Read the model definition and answer for the solid it produces. Units are mm, in the model's axes. Give positions to 0.01 mm unless a question says otherwise; leave off trailing zeros. Loops run counter-clockwise (first coordinate to the right, second up) from the corner with the lowest first, then second, coordinate; pieces in that order, holes last. Notation, with made-up numbers: (68, -23.5) - (75, -23.5) arc R29 cw to (75, 15.5) - close; hole circle Ø2 at (-18, 70). An arc over 180 degrees is marked (long way). Write each question's results on one line, items separated by ' | '. Start each with the question number.
Q1. The part is cut by section A-A, the plane x = -114.5. Write down the section's boundary in (y, z), plus the area to 3 significant figures.
Q2. Find the intervals of material crossed by line 1 (Y direction, x = -215.5, z = 2.7); line 2 (X direction, y = 172.5, z = 1.9); line 3 (Y direction, x = -101, z = 3.9), in increasing order. Write a range as from..to.
Q3. Given pin 1 (1.8 mm diameter, centred on y = 336, z = 3.5, fed in from -X); pin 2 (1.8 mm diameter, centred on x = -61, z = 3.5, fed in from -Y); pin 3 (3 mm diameter, centred on y = 123.5, z = 1.5, fed in from +X), each flat-ended and moving along its own axis, determine where each tip first touches the part or whether it passes through.
Q4. The part is cut by section B-B, the plane z = 1.8. State how many separate pieces and enclosed holes the cut face has, plus the area to 3 significant figures.
Q5. The part is cut by section D-D, the plane y = 53.5. Write down the section's boundary in (x, z), plus the area to 3 significant figures.
Q6. The part is cut by section C-C, the plane x = -172.5. Write down the section's boundary in (y, z), plus the area to 3 significant figures.
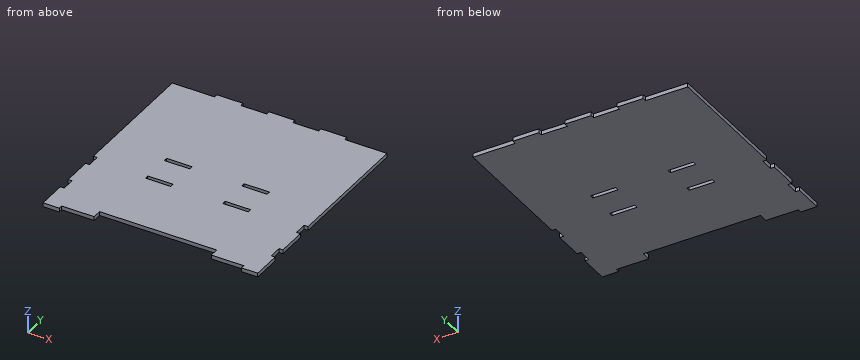
```python
from build123d import *

# Parameters (mm, degrees)
ESQUISSE1_W             = 330
ESQUISSE1_H             = 340
BOSS_EXTRU_1_DEPTH      = 6
ESQUISSE2_W             = 39
ESQUISSE2_H             = 6
ESQUISSE2_W_2           = 6
ESQUISSE2_H_2           = 20
ESQUISSE2_W_3           = 65
ESQUISSE2_W_4           = 40
ENL_V_MAT_ENCOCHE_DEPTH = 474.852297662


with BuildPart() as part:
    # Esquisse1 → Boss.-Extru.1 (new body)
    with BuildSketch(Plane.XY):
        with Locations((-165, 170)):
            Rectangle(ESQUISSE1_W, ESQUISSE1_H)
    extrude(amount=BOSS_EXTRU_1_DEPTH)

    # Esquisse2 → Enlèv. mat encoche (cut, through all)
    with BuildSketch(Plane.XY.offset(6)):
        with Locations((-224.5, 172)):
            Rectangle(ESQUISSE2_W, ESQUISSE2_H)
        with Locations((-105.5, 172)):
            Rectangle(ESQUISSE2_W, ESQUISSE2_H)
        with Locations((-327, 120)):
            Rectangle(ESQUISSE2_W_2, ESQUISSE2_H_2)
        with Locations((-327, 55)):
            Rectangle(ESQUISSE2_W_2, ESQUISSE2_H_2)
        with Locations((-3, 120)):
            Rectangle(ESQUISSE2_W_2, ESQUISSE2_H_2)
        with Locations((-3, 55)):
            Rectangle(ESQUISSE2_W_2, ESQUISSE2_H_2)
        with Locations((-224.5, 123)):
            Rectangle(ESQUISSE2_W, ESQUISSE2_H)
        with Locations((-105.5, 123)):
            Rectangle(ESQUISSE2_W, ESQUISSE2_H)
        with Locations((-297.5, 337)):
            Rectangle(ESQUISSE2_W_3, ESQUISSE2_H)
        with Locations((-205, 337)):
            Rectangle(ESQUISSE2_W_4, ESQUISSE2_H)
        with Locations((-125, 337)):
            Rectangle(ESQUISSE2_W_4, ESQUISSE2_H)
        with Locations((-32.5, 337)):
            Rectangle(ESQUISSE2_W_3, ESQUISSE2_H)
        Polygon((-305, 0), (-255, 0), (-75, 0), (-25, 0), (-25, 6), (-75, 6), (-75, 20), (-255, 20), (-255, 6), (-305, 6), align=None)
    extrude(amount=-ENL_V_MAT_ENCOCHE_DEPTH, mode=Mode.SUBTRACT)


solid = part.part
```
Check sheet entries:
1) outline: (20, 0) - (120, 0) - (120, 6) - (20, 6) - close; (126, 0) - (169, 0) - (169, 6) - (126, 6) - close; (175, 0) - (334, 0) - (334, 6) - (175, 6) - close | area: 1,810 mm^2
2) line 1: y = 20..120, 126..169, 175..334 | line 2: x = -330..-244, -205..-125, -86..0 | line 3: y = 20..120, 126..169, 175..340
3) pin 1: stops at x = -265 | pin 2: stops at y = 6 | pin 3: stops at x = -6
4) separate pieces: 1 | enclosed holes: 4 | area: 105,000 mm^2
5) outline: (-324, 0) - (-6, 0) - (-6, 6) - (-324, 6) - close | area: 1,910 mm^2
6) outline: (20, 0) - (340, 0) - (340, 6) - (20, 6) - close | area: 1,920 mm^2
